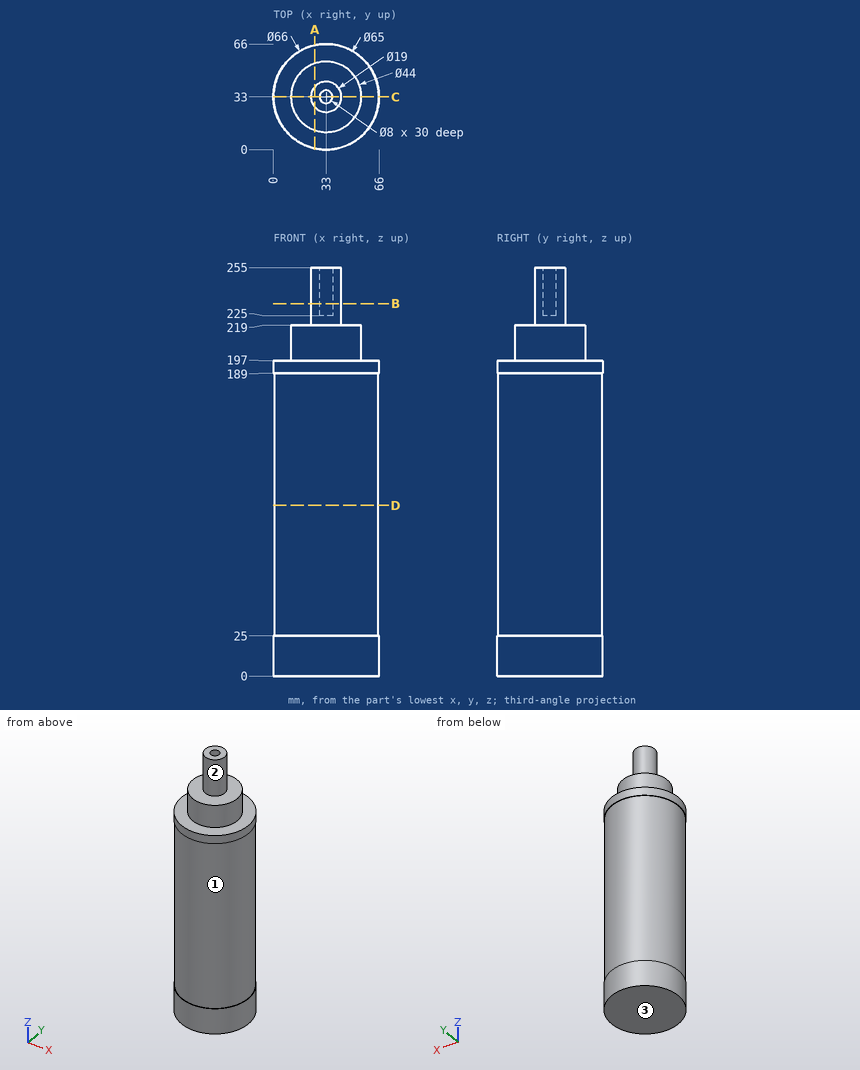
Answer from the drawing. Dimensions are ordinates in mm from the lowest x, y and z of the part. A direction names the side the tool comes from. Round coordinates to 2 decimals unless told otherwise and drop trailing zeros. Write each loop counter-clockwise with the first axis right and the second up, starting at its lowest first coordinate (ties: lowest second). Pieces come first, ordered by that corner, then holes.
1. The part is cut by section D-D, the plane z = 106.5. Determine the outline of the cut face in (x, y), then the cut area to 3 significant figures.
2. Given pin 1 Ø4 at (x, z) = (25.5, 128.5) entering from -Y; pin 2 Ø1.5 at (x, z) = (54, 178) entering from +Y; pin 3 Ø4 at (y, z) = (59, 58.5) entering from -X, each flat-ended and moving along its own axis, determine where each tip first touches the part or whether it passes through.
3. The part is cut by section A-A, the plane x = 26. Determine the outline of the cut face in (y, z).
4. The part is cut by section C-C, the plane y = 33. Determine the outline of the cut face in (x, z), then the cut area to 4 significant figures.
5. Which of the six approach directions +Z, -Z, +X, -X, +Y, -Y give full straight-line access (tool end or side, diameter ignored) to the marked faces 1, 2 and 3?
6. Straight lines are drawn through the part: L1, parallel to Y at x = 33, z = 239.75; L2, parallel to Z at x = 24, y = 28; L3, parallel to Z at x = 12, y = 10. For each, find the intervals that lie inside material, in ascending order.
7. The part is cut by section B-B, the plane z = 232.5. Determine the outline of the cut face in (x, y), then the cut area to 3 significant figures.
Values:
1. outline: circle Ø65 at (33, 33)
1. area: 3,320 mm2
2. pin 1: stops at y = 0.97
2. pin 2: stops at y = 58.42
2. pin 3: stops at x = 11.09
3. outline: (0.75, 0) - (65.25, 0) - (65.25, 25) - (64.74, 25) - (64.74, 189) - (65.25, 189) - (65.25, 197) - (53.86, 197) - (53.86, 219) - (39.42, 219) - (39.42, 255) - (26.58, 255) - (26.58, 219) - (12.14, 219) - (12.14, 197) - (0.75, 197) - (0.75, 189) - (1.26, 189) - (1.26, 25) - (0.75, 25) - close
4. outline: (0, 0) - (66, 0) - (66, 25) - (65.5, 25) - (65.5, 189) - (66, 189) - (66, 197) - (55, 197) - (55, 219) - (42.5, 219) - (42.5, 255) - (37, 255) - (37, 225) - (29, 225) - (29, 255) - (23.5, 255) - (23.5, 219) - (11, 219) - (11, 197) - (0, 197) - (0, 189) - (0.5, 189) - (0.5, 25) - (0, 25) - close
4. area: 14,250 mm2
5. face 1: none
5. face 2: +Z
5. face 3: -Z, +X, -X, +Y, -Y
6. L1: y = 23.5 to 29, 37 to 42.5
6. L2: z = 0 to 219
6. L3: z = 0 to 197
7. outline: circle Ø19 at (33, 33); hole circle Ø8 at (33, 33)
7. area: 233 mm2
